Model file for the job. Use its own axes, mm. A direction names the side the tool comes from. Coordinates: 2 decimals unless noted, no trailing zeros. Write each loop counter-clockwise with the first axis right and the second up, starting at its lowest first coordinate (ties: lowest second). Pieces come first, ordered by that corner, then holes.
Q1. Pin check, flat tips, straight feed: P1, Ø4.5, axis at x = 30, y = 0, coming from the -Z side; P2, Ø5, axis at y = 41, z = -2.5, coming from the +X side; P3, Ø3, axis at y = -2, z = -1.5, coming from the -X side. Stop position of each tip, or through.
Q2. Drill centre lines: probe 1 along X at (y, z) = (0, -5.5); probe 2 along Z at (x, y) = (-63, -35); probe 3 along Y at (x, z) = (35, -3.25). Where is each one in solid material? Low to high.
Q3. Which spindle directions (+Z, -Z, +X, -X, +Y, -Y) get a long thin tool onto all of the face, cutting with end or side? Do faces 4 (the cylindrical face through (28.25, -0.08, 1.45)), 5 (the cylindrical face through (-9.373, 71.387, 1.972)), 6 (the cylindrical face through (22.507, -0.33, -6.056)). Say none if no direction does.
Q4. Band-saw the part on A-A, the plane y = 0. Write the cut outline in (x, z).
Q5. Pull direction X, two halves, no side cores. Call faces 1 (the cylindrical face through (-9.764, -74.362, -4.93)), 2 (the flat face through (30, -2, -2)), 3 (the flat face through (-1, -1, -10)): released by +X, released by -X, zero draft, split by the parting line, or undercut.
from build123d import *

# Parameters (mm, degrees)
SKETCH_R        = 72
PAD_DEPTH       = 5
SKETCH001_R     = 75
PAD001_DEPTH    = 10
CHAMFER_SIZE    = 1
SKETCH002_R     = 1.75
POCKET_DEPTH    = 15.001
SKETCH003_R     = 7.5
POCKET001_DEPTH = 8


with BuildPart() as part:
    # Sketch → Pad (new body)
    with BuildSketch(Plane.XY):
        Circle(SKETCH_R)
    extrude(amount=PAD_DEPTH)

    # Sketch001 (on Face2 of Pad) → Pad001 (join)
    with BuildSketch(Plane(origin=(0, 0, 0), x_dir=(1, 0, 0), z_dir=(0, 0, -1))):
        Circle(SKETCH001_R)
    extrude(amount=PAD001_DEPTH)

    # Chamfer
    chamfer_edges = [part.edges().sort_by_distance(p)[0] for p in [
        (-72, 0, 5),
    ]]
    chamfer(chamfer_edges, length=CHAMFER_SIZE)

    # Sketch002 (on Face6 of Chamfer) → Pocket (cut, through all)
    with BuildSketch(Plane(origin=(0, 0, -10), x_dir=(1, 0, 0), z_dir=(0, 0, -1))):
        with Locations((30, 0)):
            Circle(SKETCH002_R)
    extrude(amount=-POCKET_DEPTH, mode=Mode.SUBTRACT)

    # Sketch003 (on Face7 of Pocket) → Pocket001 (cut)
    with BuildSketch(Plane(origin=(0, 0, -10), x_dir=(1, 0, 0), z_dir=(0, 0, -1))):
        with Locations((30, 0)):
            Circle(SKETCH003_R)
    extrude(amount=-POCKET001_DEPTH, mode=Mode.SUBTRACT)


solid = part.part
Answer sheet:
1. P1: stops at z = -2
1. P2: stops at x = 64.36
1. P3: stops at x = -75
2. probe 1: x = -75 to 22.5, 37.5 to 75
2. probe 2: z = -10 to 0
2. probe 3: y = -66.33 to -5.59, 5.59 to 66.33
3. face 4: +Z, -Z
3. face 5: +Z
3. face 6: -Z
4. outline: (-75, -10) - (22.5, -10) - (22.5, -2) - (28.25, -2) - (28.25, 5) - (-71, 5) - (-72, 4) - (-72, 0) - (-75, 0) - close; (31.75, -2) - (37.5, -2) - (37.5, -10) - (75, -10) - (75, 0) - (72, 0) - (72, 4) - (71, 5) - (31.75, 5) - close
5. face 1: split by the parting line
5. face 2: undercut
5. face 3: zero draft
